Design review of the part shown in the three views and the two pictorial views. Dimensions are in mm from the part's minimum x, y and z. A direction names the side the tool comes from. Round coordinates to 2 decimals unless told otherwise and drop trailing zeros. Loops run counter-clockwise (first coordinate to the right, second up) from the corner with the lowest first, then second, coordinate; pieces in that order, holes last.
1. Tool access review of the marked faces 1, 2 and 3: name each direction out of +Z, -Z, +X, -X, +Y, -Y from which nothing blocks a thin tool from reaching the whole face with its end or side.
2. Consider section C-C on x = 3.5. State the section outline as (y, z) points.
3. Clearance check with flat-ended pins moving along their axes: pin 1 Ø4 at (x, y) = (3, 7.5) entering from +Z; pin 2 Ø2 at (x, y) = (13, 21.5) entering from +Z; pin 3 Ø8 at (x, z) = (9.5, 28) entering from +Y; pin 4 Ø4.5 at (y, z) = (5, 5) entering from +X. State where each tip first meets the part, or that it passes through.
4. Consider section A-A on z = 5. State the section outline as (x, y) points.
5. Consider section D-D on z = 9. State the section outline as (x, y) points.
6. To check wall thickness, follow line 1 along Y through (x, z) = (2.15, 5); line 2 along Y through (x, z) = (12.25, 30.5); line 3 along X through (y, z) = (24, 6). State the ranges of each line that lie inside material, in increasing order.
7. Consider section B-B on y = 5. State the section outline as (x, z) points, then the cut area to 3 significant figures.
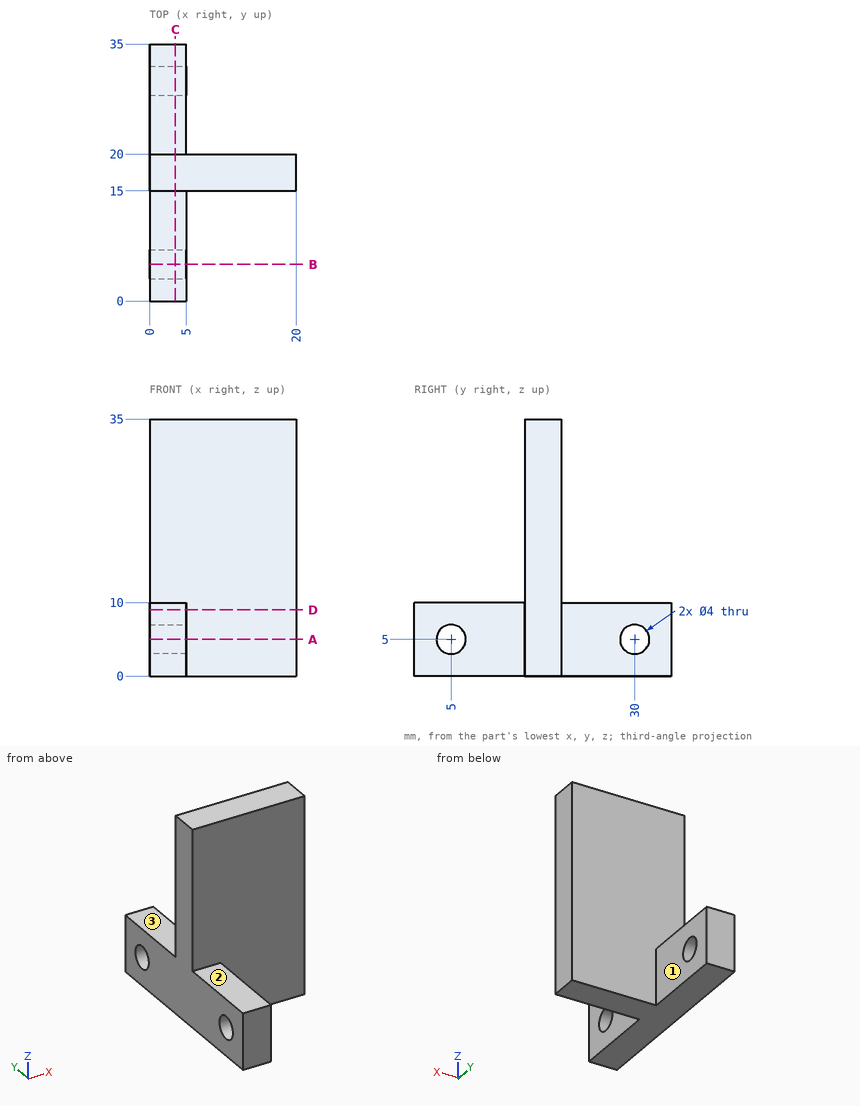
Resolved:
1. face 1: +Z, -Z, +X, +Y
1. face 2: +Z, +X, -X, -Y
1. face 3: +Z, +X, -X, +Y
2. outline: (0, 0) - (35, 0) - (35, 10) - (20, 10) - (20, 35) - (15, 35) - (15, 10) - (0, 10) - close; hole circle Ø4 at (5, 5); hole circle Ø4 at (30, 5)
3. pin 1: stops at z = 10
3. pin 2: passes through
3. pin 3: stops at y = 20
3. pin 4: stops at x = 5
4. outline: (0, 0) - (5, 0) - (5, 3) - (0, 3) - close; (0, 7) - (5, 7) - (5, 15) - (20, 15) - (20, 20) - (5, 20) - (5, 28) - (0, 28) - close; (0, 32) - (5, 32) - (5, 35) - (0, 35) - close
5. outline: (0, 0) - (5, 0) - (5, 15) - (20, 15) - (20, 20) - (5, 20) - (5, 35) - (0, 35) - close
6. line 1: y = 0 to 3, 7 to 28, 32 to 35
6. line 2: y = 15 to 20
6. line 3: x = 0 to 5
7. outline: (0, 0) - (5, 0) - (5, 3) - (0, 3) - close; (0, 7) - (5, 7) - (5, 10) - (0, 10) - close
7. area: 30.0 mm2
